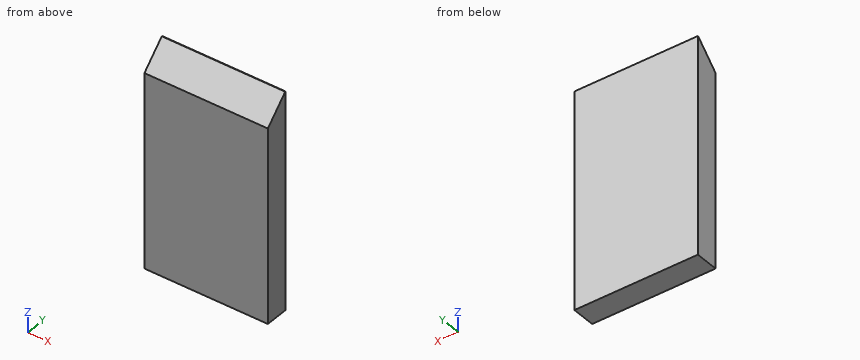
```python
from build123d import *

# Parameters (mm, degrees)
ESQUISSE1_W      = 25.8
ESQUISSE1_H      = 45.349242405
EXTRUSION1_DEPTH = 4.9
CHANFREIN2_SIZE  = 4.8


with BuildPart() as part:
    # Esquisse1 → Extrusion1 (new body)
    with BuildSketch(Plane(origin=(0, 0, 0), x_dir=(1, 0, 0), z_dir=(0, 1, 0))):
        with Locations((0, 1.325378797)):
            Rectangle(ESQUISSE1_W, ESQUISSE1_H)
    extrude(amount=EXTRUSION1_DEPTH)

    # Chanfrein2
    chanfrein2_edges = [part.edges().sort_by_distance(p)[0] for p in [
        (0, 0, 21.349242405),
    ]]
    chamfer(chanfrein2_edges, length=CHANFREIN2_SIZE)


solid = part.part
```
The listing builds one solid part. Answer for the finished solid, in the listing's coordinates (mm). Give positions to 0.01 mm unless a question says otherwise; leave off trailing zeros. Order: outer loops, then holes, each group sorted by start corner. A loop starts at its lowest first (then second) coordinate and runs counter-clockwise, first axis right, second up. Notation, with made-up numbers: (-36, 36) - (-23, 36) arc R14 cw to (-23, 55) - close; hole circle Ø8 at (-6.75, 49). An arc over 180 degrees is marked (long way). Use one line per item in the form item = value. Start each with the question number.
(1) A cutting plane is placed at C-C, the plane y = 0.95. Write down the section's boundary in (x, z), then the cut area to 3 significant figures.
(2) Consider line 1 (Z direction, x = -8.5, y = 4.35); line 2 (Z direction, x = 7.5, y = 4.25). Determine where each line is inside the solid, lowest interval first. Write a range as from..to.
(3) A flat-ended cylindrical pin translates along its axis: pin 1 Ø2 at (x, y) = (4, 3) entering from +Z. Find the tip coordinate at first contact, or state that the pin passes through.
(4) A cutting plane is placed at B-B, the plane y = 4.05. Write down the section's boundary in (x, z).
(5) A cutting plane is placed at A-A, the plane x = 4.75. Write down the section's boundary in (y, z).
Ans:
q1.outline = (-12.9, -24) - (12.9, -24) - (12.9, 17.5) - (-12.9, 17.5) - close
q1.area = 1,070 mm^2
q2.line_1 = -24..20.9
q2.line_2 = -24..20.8
q3.pin_1 = 20.55
q4.outline = (-12.9, -24) - (12.9, -24) - (12.9, 20.6) - (-12.9, 20.6) - close
q5.outline = (0, -24) - (4.9, -24) - (4.9, 21.35) - (4.8, 21.35) - (0, 16.55) - close
